Geometry: see drawing. Coordinates: mm, zero at the bounding-box minimum. A direction names the side the tool comes from. Round coordinates to 2 decimals unless told otherwise and drop trailing zeros. Loops run counter-clockwise (first coordinate to the right, second up) from the corner with the lowest first, then second, coordinate; pieces in that order, holes last. Notation, with made-up numbers: (54.25, 81.5) -> (69.25, 81.5) arc R7 cw to (69.25, 89.5) -> close; hole circle Ø3 at (66, 11.25). An arc over 180 degrees is marked (long way). Answer in a Markdown table with one row per item.
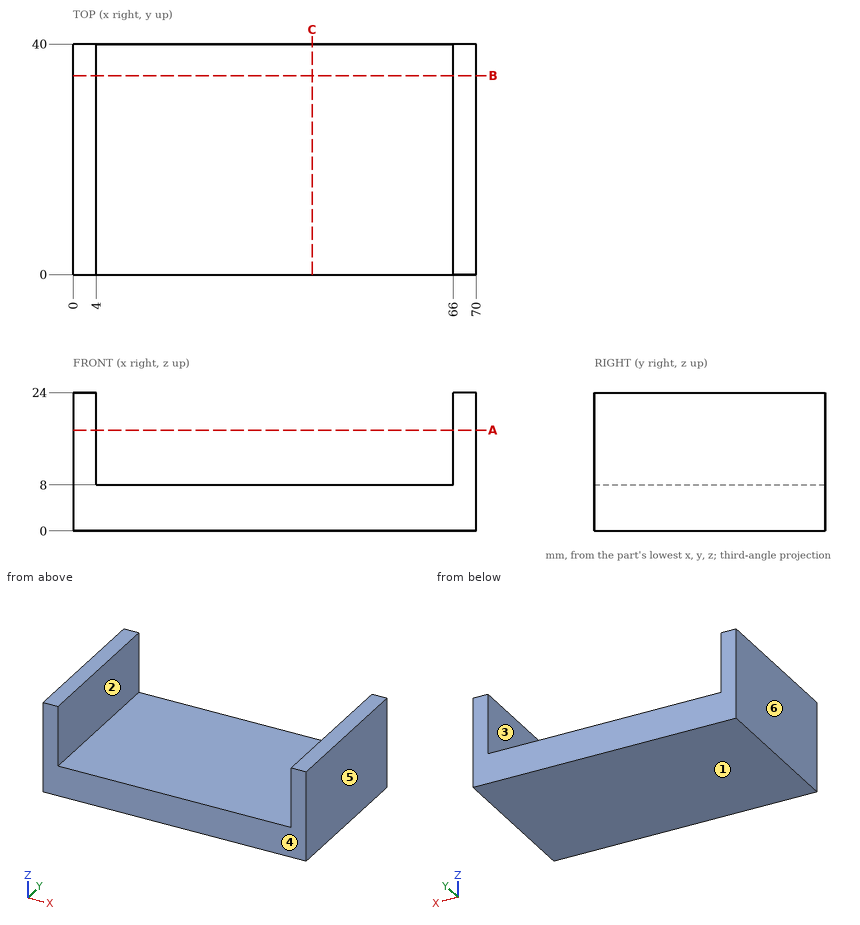
Item 1: Section query B-B, the plane y = 34.5. Output: boundary loops of the cut face in (x, z).
Ans:
| item | result |
|---|---|
| outline | (0, 0) -> (70, 0) -> (70, 24) -> (66, 24) -> (66, 8) -> (4, 8) -> (4, 24) -> (0, 24) -> close |
Item 2: Section query C-C, the plane x = 41.5. Output: boundary loops of the cut face in (y, z), and give its area (3 significant figures).
Ans:
| item | result |
|---|---|
| outline | (0, 0) -> (40, 0) -> (40, 8) -> (0, 8) -> close |
| area | 320 mm2 |
Item 3: Section query A-A, the plane z = 17.5. Output: boundary loops of the cut face in (x, y).
Ans:
| item | result |
|---|---|
| outline | (0, 0) -> (4, 0) -> (4, 40) -> (0, 40) -> close; (66, 0) -> (70, 0) -> (70, 40) -> (66, 40) -> close |
Item 4: Mould query, pull axis X, two halves, no side actions, for the marked faces 3, 4, 5 and 6. Classes: released by +X, released by -X, zero draft, split by the parting line, or undercut.
Ans:
| item | result |
|---|---|
| face 3 | undercut |
| face 4 | zero draft |
| face 5 | released by +X |
| face 6 | released by -X |
Item 5: First-contact query: P1, Ø1.5, axis at x = 33.5, y = 31, coming from the +Z side; P2, Ø1.5, axis at x = 57.5, z = 9, coming from the +Y side. Flat tips, straight axial feed; report the tip coordinate or a pass-through.
Ans:
| item | result |
|---|---|
| P1 | z = 8 |
| P2 | through |
Item 6: Ray query, L1, parallel to X at y = 33, z = 13.5; L2, parallel to Z at x = 5.5, y = 34.5. Return the intervals inside material, ascending.
Ans:
| item | result |
|---|---|
| L1 | 0 to 4, 66 to 70 |
| L2 | 0 to 8 |
Item 7: Set-up query: the marked faces 1 and 2. Return all of +Z, -Z, +X, -X, +Y, -Y with unobstructed straight access to the full face (end or side cutting, diameter ignored); none if empty.
Ans:
| item | result |
|---|---|
| face 1 | -Z, +X, -X, +Y, -Y |
| face 2 | +Z, +Y, -Y |
